from build123d import *

# Parameters (mm, degrees)
SKETCH_W        = 166
SKETCH_H        = 156
PAD_DEPTH       = 2
SKETCH001_R     = 2
POCKET_DEPTH    = 2.001
SKETCH002_R     = 3
POCKET001_DEPTH = 2.001
SKETCH003_R     = 1.5
SKETCH003_W     = 13
SKETCH003_H     = 12
POCKET002_DEPTH = 2.001


with BuildPart() as part:
    # Sketch → Pad (new body)
    with BuildSketch(Plane.XY):
        with Locations((83, 78)):
            Rectangle(SKETCH_W, SKETCH_H)
    extrude(amount=PAD_DEPTH)

    # Sketch001 (on Face6 of Pad) → Pocket (cut, through all)
    with BuildSketch(Plane.XY.offset(2)):
        with Locations((4, 152)):
            Circle(SKETCH001_R)
        with Locations((162, 152)):
            Circle(SKETCH001_R)
        with Locations((4, 4)):
            Circle(SKETCH001_R)
        with Locations((162, 4)):
            Circle(SKETCH001_R)
    extrude(amount=-POCKET_DEPTH, mode=Mode.SUBTRACT)

    # Sketch002 (on Face5 of Pocket) → Pocket001 (cut, through all)
    with BuildSketch(Plane.XY.offset(2)):
        with Locations((118, 136)):
            Circle(SKETCH002_R)
        with Locations((136, 136)):
            Circle(SKETCH002_R)
    extrude(amount=-POCKET001_DEPTH, mode=Mode.SUBTRACT)

    # Sketch003 (on Face5 of Pocket001) → Pocket002 (cut, through all)
    with BuildSketch(Plane.XY.offset(2)):
        with Locations((30, 20)):
            Circle(SKETCH003_R)
        with Locations((56, 20)):
            Circle(SKETCH003_R)
        with Locations((43, 20)):
            Rectangle(SKETCH003_W, SKETCH003_H)
    extrude(amount=-POCKET002_DEPTH, mode=Mode.SUBTRACT)


solid = part.part
CAD build for the part. Positions are in the model's coordinates, mm. Give positions to 0.01 mm unless a question says otherwise; leave off trailing zeros. Loops run counter-clockwise (first coordinate to the right, second up) from the corner with the lowest first, then second, coordinate; pieces in that order, holes last. Notation, with made-up numbers: M 15,74.5 L 21,74.5 A26 cw 21,95.5 Z; hole C -16,69.25 d6. An arc over 180 degrees is marked long. One line per question, with ' | ' between items. Start each with the question number.
1. Two-plate mould, pull along Y, no slides. Class faces 1 (the face through (160, 4, 1)), 2 (the face through (82, 79, 2)): pulls with the +Y half, pulls with the -Y half, needs draft (parallel to the pull), parting line crosses it, or undercut.
2. Saw through at C-C on y = 136. Give the cut face in (x, z), plus the area to 3 significant figures.
3. Probe L1, parallel to X at y = 136, z = 1.45; L2, parallel to Y at x = 4, z = 0.75; L3, parallel to X at y = 152, z = 1.15. List the from-to ranges inside material, lowest first. Write a range as from..to.
4. Saw through at A-A on y = 152. Give the cut face in (x, z), plus the area to 3 significant figures.
5. Saw through at B-B on x = 136. Give the cut face in (y, z).
Result sheet:
1) face 1: undercut | face 2: needs draft
2) outline: M 0,0 L 115,0 L 115,2 L 0,2 Z; M 121,0 L 133,0 L 133,2 L 121,2 Z; M 139,0 L 166,0 L 166,2 L 139,2 Z | area: 308 mm^2
3) L1: x = 0..115, 121..133, 139..166 | L2: y = 0..2, 6..150, 154..156 | L3: x = 0..2, 6..160, 164..166
4) outline: M 0,0 L 2,0 L 2,2 L 0,2 Z; M 6,0 L 160,0 L 160,2 L 6,2 Z; M 164,0 L 166,0 L 166,2 L 164,2 Z | area: 316 mm^2
5) outline: M 0,0 L 133,0 L 133,2 L 0,2 Z; M 139,0 L 156,0 L 156,2 L 139,2 Z
